Part model, mm, in its own coordinate system. Coordinates: 2 decimals unless noted, no trailing zeros. Write each loop counter-clockwise with the first axis right and the second up, starting at its lowest first coordinate (ties: lowest second). Pieces come first, ordered by that corner, then holes. Notation, with made-up numbers: (40, 4.25) -> (46, 4.25) arc R33 ccw to (46, 41.25) -> close; hole circle Ø5 at (9.25, 74). An arc over 180 degrees is marked (long way). Write item = value, one per line.
from build123d import *

# Parameters (mm, degrees)
SKETCH004_R  = 327.882384
PAD003_DEPTH = 350
FILLET_R     = 200
FILLET001_R  = 201


with BuildPart() as part:
    # Sketch004 → Pad003 (new body, symmetric)
    with BuildSketch(Plane.YZ):
        Circle(SKETCH004_R)
    extrude(amount=PAD003_DEPTH, both=True)

    # Fillet
    fillet_edges = [part.edges().sort_by_distance(p)[0] for p in [
        (-350, -327.882384, 0),
    ]]
    fillet(fillet_edges, radius=FILLET_R)

    # Fillet001
    fillet001_edges = [part.edges().sort_by_distance(p)[0] for p in [
        (350, -327.882384, 0),
    ]]
    fillet(fillet001_edges, radius=FILLET001_R)


with BuildPart() as part_1:
    # Body003 placement: moved
    add(part.part.moved(Location((-489, 0, 832))))


solid = part_1.part
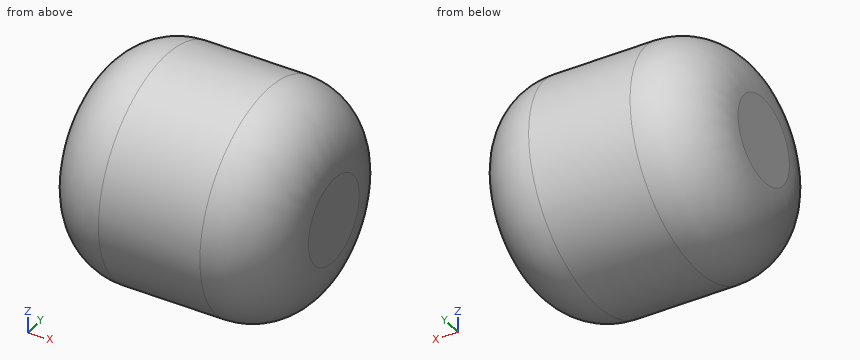
Q1. Probe line 1 (Y direction, x = -671, z = 577); line 2 (Z direction, x = -229, y = 13.5); line 3 (X direction, y = 8, z = 550). List the from-to ranges inside material, lowest first. Write a range as from..to.
Model answer:
line_1 = -201.99..201.99
line_2 = 537.86..1126.14
line_3 = -766.33..-212.31
Q2. Pin check, flat tips, straight feed: pin 1 (5 mm diameter, centred on x = -757.5, z = 829, fed in from +Y); pin 2 (5 mm diameter, centred on x = -422.5, z = 981.5, fed in from +Y); pin 3 (4 mm diameter, centred on y = 63, z = 573.5, fed in from -X). Stop position of each tip, or through.
Model answer:
pin_1 = 290.79
pin_2 = 293.08
pin_3 = -785.47
Q3. Saw through at A-A on x = -396. Give the cut face in (y, z).
Model answer:
outline = circle Ø655.76 at (0, 832)
